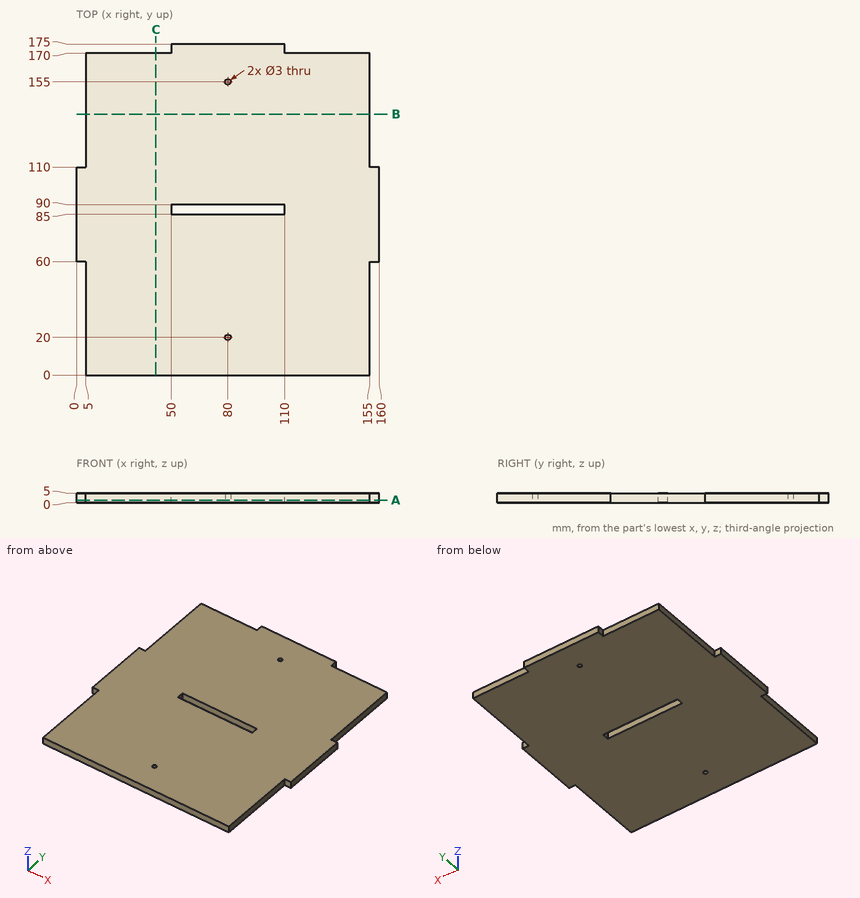
Print and shaded views of the part. All mm, measured from the part's lowest x, y and z. Coordinates: 2 decimals unless noted, no trailing zeros. Order: outer loops, then holes, each group sorted by start corner. A loop starts at its lowest first (then second) coordinate and runs counter-clockwise, first axis right, second up. Notation, with made-up numbers: (31, 54.5) -> (88, 54.5) arc R11 ccw to (88, 73.5) -> close; hole circle Ø1 at (21, -7). An arc over 180 degrees is marked (long way). Use one line per item in the form item = value. Start each with the question number.
1) Band-saw the part on C-C on x = 42. Give the cut face in (y, z), then the cut area to 3 significant figures.
2) Band-saw the part on A-A on z = 1.3. Give the cut face in (x, y), then the cut area to 3 significant figures.
3) Band-saw the part on B-B on y = 138. Give the cut face in (x, z), then the cut area to 3 significant figures.
4) Drill centre lines: L1, parallel to Y at x = 80, z = 1.7; L2, parallel to X at y = 20, z = 1.3; L3, parallel to Y at x = 73, z = 3.55. Where is each one in solid material? Low to high. Write a range as [from, to].
5) Drop flat-ended pins along their axis: pin 1 (1.5 mm diameter, centred on x = 2, z = 3, fed in from +Y); pin 2 (2.5 mm diameter, centred on y = 148, z = 2, fed in from +X); pin 3 (1.5 mm diameter, centred on x = 2.5, z = 1.5, fed in from -Y). Give the stop position or say it passes through.
Entries:
q1.outline = (0, 0) -> (170, 0) -> (170, 5) -> (0, 5) -> close
q1.area = 850 mm2
q2.outline = (0, 60) -> (5, 60) -> (5, 0) -> (155, 0) -> (155, 60) -> (160, 60) -> (160, 110) -> (155, 110) -> (155, 170) -> (110, 170) -> (110, 175) -> (50, 175) -> (50, 170) -> (5, 170) -> (5, 110) -> (0, 110) -> close; hole (50, 85) -> (110, 85) -> (110, 90) -> (50, 90) -> close; hole circle Ø3 at (80, 20); hole circle Ø3 at (80, 155)
q2.area = 26,000 mm2
q3.outline = (5, 0) -> (155, 0) -> (155, 5) -> (5, 5) -> close
q3.area = 750 mm2
q4.L1 = [0, 18.5], [21.5, 85], [90, 153.5], [156.5, 175]
q4.L2 = [5, 78.5], [81.5, 155]
q4.L3 = [0, 85], [90, 175]
q5.pin_1 = 110
q5.pin_2 = 155
q5.pin_3 = 60
